Work out the finished part from the listing and answer in its coordinate system (mm). Coordinates: 2 decimals unless noted, no trailing zeros. Write each loop counter-clockwise with the first axis right and the second up, starting at its lowest first coordinate (ties: lowest second). Pieces come first, ordered by that corner, then holes. Notation, with made-up numbers: (49.5, -28) - (96.5, -28) arc R20 cw to (96.5, -5) - close; hole circle Ø4 at (21, 80.25). An arc over 180 degrees is marked (long way). Use one line per item in the form item = value. Start each with the question number.
Item 1: A cutting plane is placed at A-A (y = 58.5). Write down the section's boundary in (x, z) (3 decimals), then the cut area to 3 significant figures.
Item 2: Consider probe 1 along Z at (x, y) = (77, 137); probe 2 along X at (y, z) = (40.5, 1.05); probe 3 along Y at (x, z) = (77, 3.6). Determine where each line is inside the solid, lowest interval first.
Item 3: Determine the mould class of faces 1 (the cylindrical face through (-16.49, 31.51, 2.01)), 2 (the flat face through (59, 0, 2)), 3 (the flat face through (-10.14, 17.56, 2.46)), 4 (the cylindrical face through (-0.252, 3.395, 0.835)) for opening direction X: released by +X, released by -X, zero draft, split by the parting line, or undercut.
Item 4: Given pin 1 (2 mm diameter, centred on x = 113.5, z = 2.5, fed in from +Y), flat-ended and moving along its own axis, determine where the tip first touches the part or whether it passes through.
Item 5: A cutting plane is placed at B-B (x = 111). Write down the section's boundary in (y, z).
from build123d import *

# Parameters (mm, degrees)
BOSS_EXTRUDE1_DEPTH = 5
SKETCH3_R           = 1.5
CUT_EXTRUDE1_DEPTH  = 3
SKETCH4_R           = 1.5
CUT_EXTRUDE2_DEPTH  = 3
SKETCH5_R           = 1.5
CUT_EXTRUDE3_DEPTH  = 3


with BuildPart() as part:
    # Sketch1 → Boss-Extrude1 (new body)
    with BuildSketch(Plane.XY):
        Polygon((0, 0), (120, 0), (140, 34.641016151), (80, 138.564064606), (40, 138.564064606), (-20, 34.641016151), align=None)
    extrude(amount=BOSS_EXTRUDE1_DEPTH)

    # Sketch3 → Cut-Extrude1 (cut)
    with BuildSketch(Plane(origin=(0, 0, 0), x_dir=(0, 0, 1), z_dir=(-0.866025404, -0.5, 0))):
        with Locations((2.333426925, 37)):
            Circle(SKETCH3_R)
        with Locations((2.333426925, 3)):
            Circle(SKETCH3_R)
    extrude(amount=-CUT_EXTRUDE1_DEPTH, mode=Mode.SUBTRACT)

    # Sketch4 → Cut-Extrude2 (cut)
    with BuildSketch(Plane(origin=(90, -51.961524227, 0), x_dir=(0, 0, -1), z_dir=(0.866025404, -0.5, 0))):
        with Locations((-2.085466333, 63)):
            Circle(SKETCH4_R)
        with Locations((-2.085466333, 97)):
            Circle(SKETCH4_R)
    extrude(amount=-CUT_EXTRUDE2_DEPTH, mode=Mode.SUBTRACT)

    # Sketch5 → Cut-Extrude3 (cut)
    with BuildSketch(Plane(origin=(0, 138.564064606, 0), x_dir=(1, 0, 0), z_dir=(0, 1, 0))):
        with Locations((77, -2.397088123)):
            Circle(SKETCH5_R)
        with Locations((43, -2.397088123)):
            Circle(SKETCH5_R)
    extrude(amount=-CUT_EXTRUDE3_DEPTH, mode=Mode.SUBTRACT)


solid = part.part
Answer:
q1.outline = (-6.225, 0) - (126.225, 0) - (126.225, 5) - (-6.225, 5) - close
q1.area = 662 mm²
q2.probe_1 = 0 to 0.9, 3.9 to 5
q2.probe_2 = -16.62 to 136.62
q2.probe_3 = 0 to 135.56
q3.face_1 = undercut
q3.face_2 = zero draft
q3.face_3 = released by -X
q3.face_4 = undercut
q4.pin_1 = 82.27
q5.outline = (0, 0) - (84.87, 0) - (84.87, 5) - (0, 5) - close
